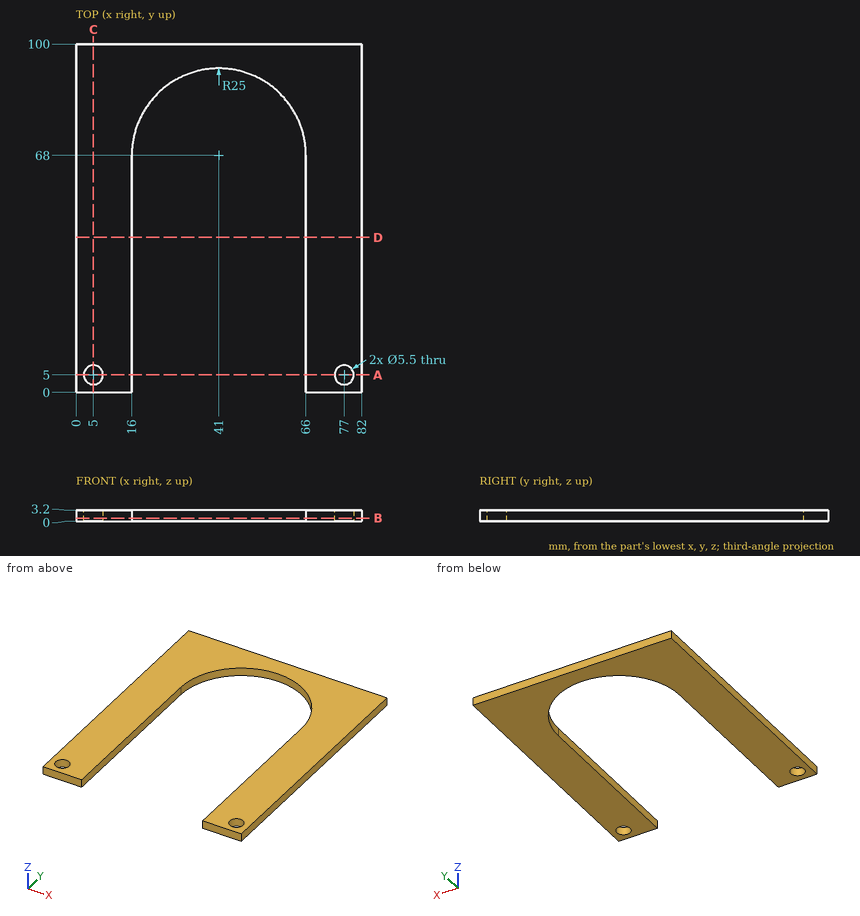
Design review of the part shown in the three views and the two pictorial views. Dimensions are in mm from the part's minimum x, y and z. Round coordinates to 2 decimals unless told otherwise and drop trailing zeros. Loops run counter-clockwise (first coordinate to the right, second up) from the corner with the lowest first, then second, coordinate; pieces in that order, holes last. Notation, with made-up numbers: (-31.5, 71) - (-14.5, 71) arc R31 ccw to (-14.5, 106) - close; hole circle Ø5 at (63.25, 7.25). An arc over 180 degrees is marked (long way). One line per item, written item: value. Start each with the question number.
Item 1: Take a section at A-A (y = 5). Give the boundary of the cut face in (x, z).
Item 2: For L1, parallel to Y at x = 5, z = 1.95; L2, parallel to X at y = 63.5, z = 2.85; L3, parallel to X at y = 90, z = 2.5, list the stretches that pass through material, from the lowest coordinate up.
Item 3: Take a section at B-B (z = 1). Give the boundary of the cut face in (x, y), plus the area to 3 significant figures.
Item 4: Take a section at D-D (y = 44.5). Give the boundary of the cut face in (x, z).
Item 5: Take a section at C-C (x = 5). Give the boundary of the cut face in (y, z), plus the area to 3 significant figures.
Item 6: Clearance check with flat-ended pins moving along their axes: pin 1 Ø1.5 at (x, z) = (63, 0.5) entering from -Y; pin 2 Ø6 at (x, y) = (62, 20) entering from -Z; pin 3 Ø6.5 at (x, y) = (77, 5) entering from +Z. State where each tip first meets the part, or that it passes through.
Answer below:
1. outline: (0, 0) - (2.25, 0) - (2.25, 3.2) - (0, 3.2) - close; (7.75, 0) - (16, 0) - (16, 3.2) - (7.75, 3.2) - close; (66, 0) - (74.25, 0) - (74.25, 3.2) - (66, 3.2) - close; (79.75, 0) - (82, 0) - (82, 3.2) - (79.75, 3.2) - close
2. L1: y = 0 to 2.25, 7.75 to 100
2. L2: x = 0 to 16, 66 to 82
2. L3: x = 0 to 29.13, 52.87 to 82
3. outline: (0, 0) - (16, 0) - (16, 68) arc R25 cw to (66, 68) - (66, 0) - (82, 0) - (82, 100) - (0, 100) - close; hole circle Ø5.5 at (5, 5); hole circle Ø5.5 at (77, 5)
3. area: 3,770 mm2
4. outline: (0, 0) - (16, 0) - (16, 3.2) - (0, 3.2) - close; (66, 0) - (82, 0) - (82, 3.2) - (66, 3.2) - close
5. outline: (0, 0) - (2.25, 0) - (2.25, 3.2) - (0, 3.2) - close; (7.75, 0) - (100, 0) - (100, 3.2) - (7.75, 3.2) - close
5. area: 302 mm2
6. pin 1: stops at y = 78.37
6. pin 2: passes through
6. pin 3: stops at z = 3.2
